Can you work these out from the model? Positions are in its coordinate system, mm. A direction names the side the tool comes from. Coordinates: 2 decimals unless noted, no trailing zeros. Order: outer loops, then holes, each group sorted by start corner. A loop starts at its lowest first (then second) coordinate and runs counter-clockwise, first axis right, second up. Notation, with made-up numbers: (27.5, 73) -> (50.5, 73) arc R25 ccw to (50.5, 109) -> close; hole circle Ø4 at (-23.75, 28.25). An arc over 180 degrees is marked (long way). Write item = value, one per line. Start each with the question number.
Autodesk Inventor part; units mm, degrees
ref_plane "Work Plane1" through (0, 0, 9.2) normal (0, 0, 1) x (1, 0, 0)
ref_plane "YZ Plane" through (0, 0, 0) normal (1, 0, 0) x (0, 1, 0)
ref_plane "XZ Plane" through (0, 0, 0) normal (0, 1, 0) x (-1, 0, 0)
sketch "スケッチ1" plane through (0, 0, 0) normal (0, 0, 1) x (1, 0, 0)
  line L0 (-15, -15) -> (15, -15)
  line L1 (15, -15) -> (15, 15)
  line L2 (15, 15) -> (-15, 15)
  line L3 (-15, 15) -> (-15, -15)
  line L4 (-15, -15) -> (15, 15) construction
  line L5 (15, -15) -> (-15, 15) construction
  line L6 (-15, 0) -> (15, 0) construction
  line L7 (0, 15) -> (0, -15) construction
  line L8 (-13.14, 13.14) -> (13.14, 13.14) construction
  line L9 (13.14, 13.14) -> (13.14, -13.14) construction
  line L10 (13.14, -13.14) -> (-13.14, -13.14) construction
  line L11 (-13.14, -13.14) -> (-13.14, 13.14) construction
  line L12 (-13.14, 13.14) -> (13.14, -13.14) construction
  line L13 (13.14, 13.14) -> (-13.14, -13.14) construction
  circle A0 centre (0, 0) radius 7
  line L14 (-7, 8) -> (7, 8)
  line L15 (8, 7) -> (8, -7)
  line L16 (7, -8) -> (-7, -8)
  line L17 (-8, -7) -> (-8, 7)
  line L18 (-8, 8) -> (8, -8) construction
  line L19 (8, 8) -> (-8, -8) construction
  arc A1 (-8, -7) -> (-7, -8) centre (-7, -7) ccw
  arc A2 (7, -8) -> (8, -7) centre (7, -7) ccw
  arc A3 (8, 7) -> (7, 8) centre (7, 7) ccw
  arc A4 (-7, 8) -> (-8, 7) centre (-7, 7) ccw
  arc A5 (-2, -10) -> (2, -10) centre (0, -10) ccw
  line L20 (-2, -10) -> (-2, -8)
  line L21 (2, -10) -> (2, -8)
  arc A6 (2, 10) -> (-2, 10) centre (0, 10) ccw
  line L22 (-2, 10) -> (-2, 8)
  line L23 (2, 10) -> (2, 8)
  circle A7 centre (-13.14, -13.14) radius 1.1
  circle A8 centre (13.14, -13.14) radius 1.1
  circle A9 centre (-13.14, 13.14) radius 1.1
  circle A10 centre (13.14, 13.14) radius 1.1
  circle A11 centre (-13.14, -13.14) radius 2 construction
  circle A12 centre (13.14, -13.14) radius 2 construction
  circle A13 centre (-13.14, 13.14) radius 2 construction
  circle A14 centre (13.14, 13.14) radius 2 construction
  arc A15 (-10.1414, -13.05) -> (-13.05, -10.1414) centre (-13.14, -13.14) ccw
  line L24 (-14.99, -8.1423) -> (-14.99, 8.1423)
  line L25 (-8.1423, -14.99) -> (8.1423, -14.99)
  arc A16 (-14.99, -8.1423) -> (-13.05, -10.1414) centre (-12.99, -8.1423) ccw
  arc A17 (-10.1414, -13.05) -> (-8.1423, -14.99) centre (-8.1423, -12.99) ccw
  arc A18 (-13.05, 10.1414) -> (-10.1414, 13.05) centre (-13.14, 13.14) ccw
  line L26 (-8.1423, 14.99) -> (8.1423, 14.99)
  arc A19 (-13.05, 10.1414) -> (-14.99, 8.1423) centre (-12.99, 8.1423) ccw
  arc A20 (-8.1423, 14.99) -> (-10.1414, 13.05) centre (-8.1423, 12.99) ccw
  arc A21 (13.05, -10.1414) -> (10.1414, -13.05) centre (13.14, -13.14) ccw
  line L27 (14.99, -8.1423) -> (14.99, 8.1423)
  arc A22 (13.05, -10.1414) -> (14.99, -8.1423) centre (12.99, -8.1423) ccw
  arc A23 (8.1423, -14.99) -> (10.1414, -13.05) centre (8.1423, -12.99) ccw
  arc A24 (14.99, 8.1423) -> (13.05, 10.1414) centre (12.99, 8.1423) ccw
  arc A25 (10.1414, 13.05) -> (13.05, 10.1414) centre (13.14, 13.14) ccw
  arc A26 (10.1414, 13.05) -> (8.1423, 14.99) centre (8.1423, 12.99) ccw
  point P0 (-10.7783, -14.99)
  point P1 (-14.99, -10.7783)
  point P2 (-8, -2.8723)
  point P3 (-8, 2.8723)
  point P4 (-2.8723, 8)
  point P5 (-2, 8.2614)
  point P6 (2, 8.2614)
  point P7 (2.8723, 8)
  point P8 (8, 2.8723)
  point P9 (8, -2.8723)
  point P10 (2.8723, -8)
  point P11 (2, -8.2614)
  point P12 (-2, -8.2614)
  point P13 (-2.8723, -8)
  point P14 (8.1423, 14.99)
  point P15 (14.99, 8.1423)
  dimension "d0" = 30
  dimension "d1" = 30
  dimension "d2" = 26.28
  dimension "d3" = 26.28
  dimension "d4" = 14
  dimension "d5" = 16
  dimension "d6" = 16
  dimension "d7" = 1
  dimension "d8" = 20
  dimension "d9" = 2
  dimension "d10" = 2.2
  dimension "d11" = 4
  dimension "d12" = 2
  dimension "d13" = 3
  dimension "d14" = 0.01
  dimension "d15" = 0.01
extrude "押し出し1" add sketch "スケッチ1" along normal blind 9.2 contours L3 L2 L1 L0 | A0 | L14 A3 L15 A2 L16 A1 L17 A4 | L22 A6 L23 L14 | L16 L21 A5 L20 | A15 A16 L24 A19 A18 A20 L26 A26 A25 A24 L27 A22 A21 A23 L25 A17
extrude "押し出し2" cut sketch "スケッチ1" along normal blind 7.6 contours L3 L2 L1 L0 | A7 | A8 | A9 | A10
extrude "押し出し3" add sketch "スケッチ1" along normal blind 1.6 contours L3 L2 L1 L0
extrude "押し出し4" add sketch "スケッチ1" along normal blind 12.7 contours A0 | L14 A3 L15 A2 L16 A1 L17 A4 | L22 A6 L23 L14 | L16 L21 A5 L20
extrude "押し出し5" add sketch "スケッチ1" along normal blind 22.2 contours A0
sketch "Sketch3" plane through (0, 0, 22.2) normal (0, 0, 1) x (1, 0, 0)
  point P0 (0, 0)
  point P1 (0, 0)
hole "Hole1" at (0, 0, 22.2) direction (0, 0, -1) diameter 10.106 depth 10
ref_plane "Work Plane1" through (0, 0, 9.2) normal (0, 0, 1) x (1, 0, 0)
equation "\"d1\" = d0"
equation "\"d3\" = d2"
equation "\"d6\" = d5"
equation "\"d15\" = d14"
properties part number "e-CAM50_CUONX"
(1) If I drill on L1, parallel to X at y = 13.14, z = 8.45; L2, parallel to Y at x = 0, z = 19, over which ranges is the centre line in solid material (lowest first)? Write a range as from..to.
(2) Imagine slicing it at A-A (z = 10.5). Write out the boundary of the cut face in (x, y).
(3) Imagine slicing it at D-D (z = 4). Write out the boundary of the cut face in (x, y), plus the area to 3 significant figures.
(4) For faces 1 (the face through (5, -8, 11)), 2 (the face through (14.41, 9.55, 4.56)), 3 (the face through (-10, 0, 9.2)), 4 (the face through (-7.699, -7.715, 10.926)), which set-ups out of +Z, -Z, +X, -X, +Y, -Y let a thin tool reach every point of the face, with its end or its side?
(5) Thinking about a two-plate mould opening in X: for faces 5 (the face through (0, 0, 12.2)), 6 (the face through (0, 12, 11)), 7 (the face through (-14.41, -9.55, 4.56)), which applies, +X half, -X half, draft (parallel to the pull), parting line (faces both ways), or undercut?
(6) For P1, Ø1.8, axis at x = 4, z = 11, coming from the -Y side; P2, Ø6.5, axis at y = 2.5, z = 5, coming from the +X side; P3, Ø8, axis at x = 4.5, z = 18.5, coming from the +Y side; P4, Ø5, axis at x = 0.5, z = 4.5, coming from the -Y side, each with a flat end and sliding along its axis, tell me the tip position at first contact or that it passes through.
Result set:
q1.L1 = -15..-14.24, -12.04..12.04, 14.24..15
q1.L2 = -7..-5.05, 5.05..7
q2.outline = (-8, -7) arc R1 ccw to (-7, -8) -> (-2, -8) -> (-2, -10) arc R2 ccw to (2, -10) -> (2, -8) -> (7, -8) arc R1 ccw to (8, -7) -> (8, 7) arc R1 ccw to (7, 8) -> (2, 8) -> (2, 10) arc R2 ccw to (-2, 10) -> (-2, 8) -> (-7, 8) arc R1 ccw to (-8, 7) -> close
q3.outline = (-14.99, -8.14) arc R2 ccw to (-13.05, -10.14) arc R3 cw to (-10.14, -13.05) arc R2 ccw to (-8.14, -14.99) -> (8.14, -14.99) arc R2 ccw to (10.14, -13.05) arc R3 cw to (13.05, -10.14) arc R2 ccw to (14.99, -8.14) -> (14.99, 8.14) arc R2 ccw to (13.05, 10.14) arc R3 cw to (10.14, 13.05) arc R2 ccw to (8.14, 14.99) -> (-8.14, 14.99) arc R2 ccw to (-10.14, 13.05) arc R3 cw to (-13.05, 10.14) arc R2 ccw to (-14.99, 8.14) -> close
q3.area = 806 mm2
q4.face_1 = +Z, +X, -Y
q4.face_2 = +X, +Y
q4.face_3 = +Z
q4.face_4 = +Z, -X, -Y
q5.face_5 = undercut
q5.face_6 = parting line
q5.face_7 = -X half
q6.P1 = -8
q6.P2 = 15
q6.P3 = 6.98
q6.P4 = -14.99
